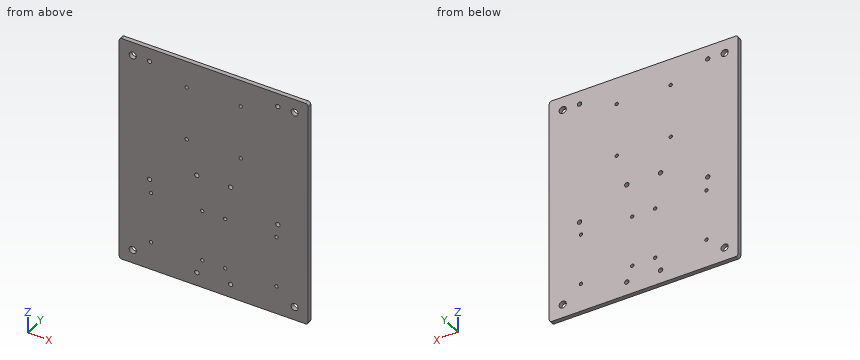
from build123d import *

# Parameters (mm, degrees)
SKETCH1_W             = 140
SKETCH1_H             = 170
BOSS_EXTRUDE1_DEPTH   = 3.175
M3X0_5_TAPPED_HOLE1_D = 2.5
M3_CLEARANCE_HOLE1_D  = 3.2
M4X0_7_TAPPED_HOLE2_D = 3.3
M5_CLEARANCE_HOLE2_D  = 5.3
FILLET1_R             = 2


with BuildPart() as part:
    # Sketch1 → Boss-Extrude1 (new body)
    with BuildSketch(Plane(origin=(0, 0, 0), x_dir=(1, 0, 0), z_dir=(0, 1, 0))):
        Rectangle(SKETCH1_W, SKETCH1_H)
    extrude(amount=BOSS_EXTRUDE1_DEPTH)

    # M3x0.5 Tapped Hole1 (through all)
    with Locations(Plane(origin=(0, 3.175, 0), x_dir=(1, 0, 0), z_dir=(0, 1, 0))):
        with Locations((-46.5, 64), (-46.5, 26), (-8.5, 26), (-8.5, 64), (8.5, 64), (46.5, 64), (8.5, 26), (46.5, 26), (-20, -25), (20, -25), (-20, -65), (20, -65)):
            Hole(M3X0_5_TAPPED_HOLE1_D / 2)

    # M3 Clearance Hole1 (through all)
    with Locations(Plane(origin=(0, 3.175, 0), x_dir=(1, 0, 0), z_dir=(0, 1, 0))):
        with Locations((-47.5, 16), (47.5, 16), (47.5, -75), (-47.5, -75)):
            Hole(M3_CLEARANCE_HOLE1_D / 2)

    # M4x0.7 Tapped Hole2 (through all)
    with Locations(Plane(origin=(0, 3.175, 0), x_dir=(1, 0, 0), z_dir=(0, 1, 0))):
        with Locations((-12.5, 75), (12.5, 75), (-12.5, 0), (12.5, 0)):
            Hole(M4X0_7_TAPPED_HOLE2_D / 2)

    # M5 Clearance Hole2 (through all)
    with Locations(Plane(origin=(0, 3.175, 0), x_dir=(1, 0, 0), z_dir=(0, 1, 0))):
        with Locations((-60, 75), (60, 75), (-60, -75), (60, -75)):
            Hole(M5_CLEARANCE_HOLE2_D / 2)

    # Fillet1
    fillet1_edges = [part.edges().sort_by_distance(p)[0] for p in [
        (70, 1.5875, 85),
        (-70, 1.5875, 85),
        (-70, 1.5875, -85),
        (70, 1.5875, -85),
    ]]
    fillet(fillet1_edges, radius=FILLET1_R)


solid = part.part
The model under review builds one solid part; all positions refer to its coordinate system, in mm. Round coordinates to 2 decimals unless told otherwise and drop trailing zeros. Order: outer loops, then holes, each group sorted by start corner. A loop starts at its lowest first (then second) coordinate and runs counter-clockwise, first axis right, second up. Notation, with made-up numbers: (10, 73) -> (22, 73) arc R28 ccw to (22, 109) -> close; hole circle Ø2 at (-20, 78.5). An arc over 180 degrees is marked (long way). Return JSON: item names as keys, results as strings.
1. Insertion check: P1, Ø5, axis at x = 60, z = -75, coming from the -Y side; P2, Ø4, axis at x = -12.5, z = -75, coming from the +Y side (3 decimals). Each pin has a flat end and moves straight along its axis. Give the tip position at first contact, or say it passes through.
Answer block:
{"P1": "passes through", "P2": "stops at y = 3.175"}
2. Take a section at A-A (x = -60). Write out the cut boundary in (y, z) (3 decimals), then the cut area to 3 significant figures.
Answer block:
{"outline": "(0, -85) -> (3.175, -85) -> (3.175, -77.65) -> (0, -77.65) -> close; (0, -72.35) -> (3.175, -72.35) -> (3.175, 72.35) -> (0, 72.35) -> close; (0, 77.65) -> (3.175, 77.65) -> (3.175, 85) -> (0, 85) -> close", "area": "506 mm²"}
3. For L1, parallel to Z at x = 60, y = 1.65; L2, parallel to X at y = 1.15, z = 25; L3, parallel to Z at x = -8.5, y = 1, list the stretches that pass through material, from the lowest coordinate up. Write a range as [from, to].
Answer block:
{"L1": "z = [-85, -77.65], [-72.35, 72.35], [77.65, 85]", "L2": "x = [-70, -21.25], [-18.75, 18.75], [21.25, 70]", "L3": "z = [-85, -65.25], [-62.75, -27.25], [-24.75, 85]"}
